Here's the drawing with two shaded views (mm, measured from the low corner). I have some questions. A direction names the side the tool comes from. Give positions to 0.01 mm unless a question says otherwise; leave off trailing zeros. Loops run counter-clockwise (first coordinate to the right, second up) from the corner with the lowest first, then second, coordinate; pieces in that order, holes last. Notation, with made-up numbers: (-8, -12.5) - (25, -12.5) arc R29 ccw to (25, 9.5) - close; hole circle Ø9 at (70, -27.5). An arc over 180 degrees is marked (long way). Use one line per item in the form item = value.
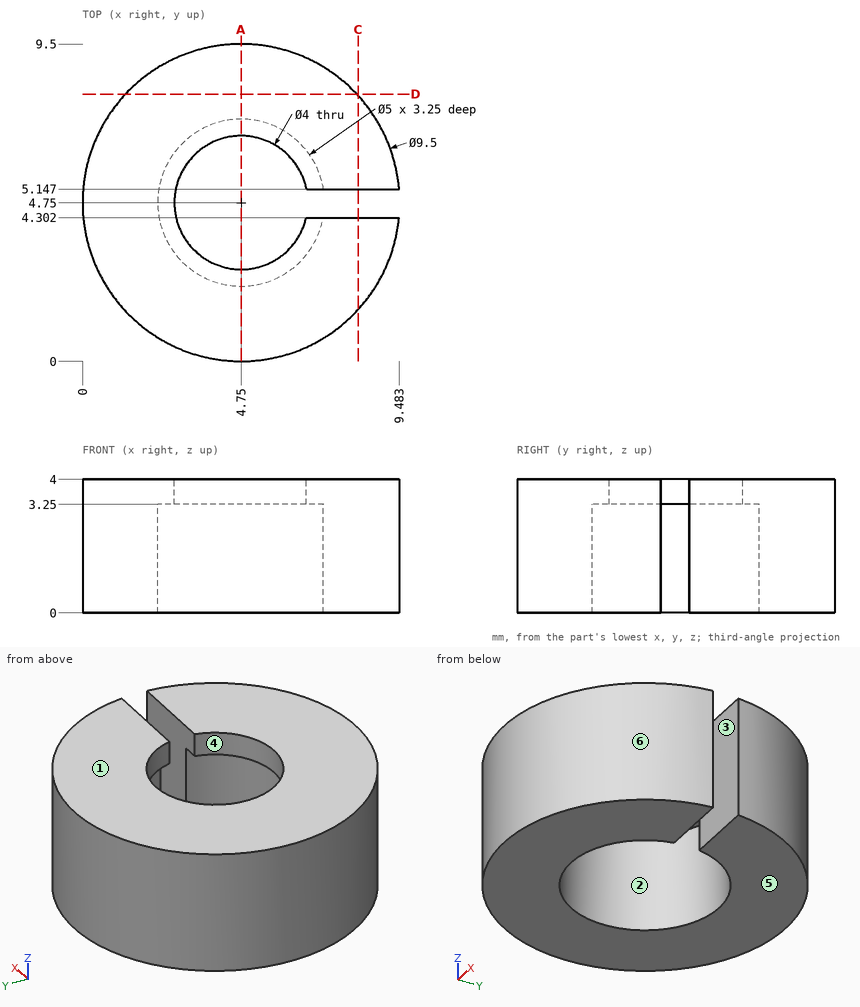
(1) If we section it at D-D (y = 8): List the corners of the cut face in (x, z) for me, plus the area to 3 significant figures.
Geometry says:
outline = (1.29, 0) - (8.21, 0) - (8.21, 4) - (1.29, 4) - close
area = 27.7 mm²
(2) If we section it at C-C (x = 8.25): List the corners of the cut face in (y, z) for me.
Geometry says:
outline = (1.54, 0) - (4.3, 0) - (4.3, 4) - (1.54, 4) - close; (5.15, 0) - (7.96, 0) - (7.96, 4) - (5.15, 4) - close
(3) Thinking about a two-plate mould opening in X: for the marked faces 4, 5 and 6, which applies, pulls with the +X half, pulls with the -X half, needs draft (parallel to the pull), parting line crosses it, or undercut?
Geometry says:
face_4 = undercut
face_5 = needs draft
face_6 = parting line crosses it
(4) If I drill on probe 1 along Y at (x, z) = (4.75, 3.6); probe 2 along Y at (x, z) = (4.75, 1.9); probe 3 along X at (y, z) = (4.75, 3), over which ranges is the centre line in solid material (lowest first)?
Geometry says:
probe_1 = 0 to 2.75, 6.75 to 9.5
probe_2 = 0 to 2.25, 7.25 to 9.5
probe_3 = 0 to 2.25
(5) For the marked faces 1, 2 and 3, which set-ups out of +Z, -Z, +X, -X, +Y, -Y let a thin tool reach every point of the face, with its end or its side?
Geometry says:
face_1 = +Z, +X, -X, +Y, -Y
face_2 = -Z
face_3 = +Z, -Z, +X
(6) If we section it at A-A (x = 4.75): List the corners of the cut face in (y, z) for me.
Geometry says:
outline = (0, 0) - (2.25, 0) - (2.25, 3.25) - (2.75, 3.25) - (2.75, 4) - (0, 4) - close; (6.75, 3.25) - (7.25, 3.25) - (7.25, 0) - (9.5, 0) - (9.5, 4) - (6.75, 4) - close
(7) For P1, Ø2, axis at y = 2.5, z = 3, coming from the -X side; P2, Ø1.4, axis at x = 8, z = 1.5, coming from the +Y side; P3, Ø1, axis at y = 1, z = 3.5, coming from the +X side (1 decimal), each with a flat end and sliding along its axis, tell me the tip position at first contact or that it passes through.
Geometry says:
P1 = 0.17
P2 = 8.76
P3 = 8.2
